Could you check a few things on this model? Use its own coordinates, in mm. A direction names the side the tool comes from. Coordinates: 2 decimals unless noted, no trailing zeros. Order: outer loops, then holes, each group sorted by start corner. A loop starts at its lowest first (then second) coordinate and runs counter-clockwise, first axis right, second up. Notation, with made-up numbers: (22.25, 33) -> (46.25, 33) arc R25 ccw to (46.25, 45) -> close; hole circle Ø11 at (-12.75, 86). An arc over 180 degrees is marked (long way). Use a Markdown table: item, result. Add a question column.
1) Will this pin go through, and if not, where does the flat tip stop? pin 1 Ø3 at (x, z) = (-2, -4.5) entering from -Y.
2) If we section it at C-C (z = 3.75): Write out the boundary of the cut face in (x, y), plus the area to 3 significant figures.
3) If I drill on L1, parallel to Y at x = 0.15, z = 0.5; L2, parallel to X at y = -0.1, z = 7; L3, parallel to Y at x = -1.7, z = 5.75, over which ranges is the centre line in solid material (lowest first)? Write a range as [from, to].
4) Which directions (+Z, -Z, +X, -X, +Y, -Y) give clear straight access to the entire face, cutting with the end or side of a thin tool? Please do faces 1 (the cylindrical face through (0, 2, 0)), 2 (the flat face through (1, -2, -10)), 3 (the flat face through (-1, 2, 10)).
5) Thinking about a two-plate mould opening in Z: for faces 4 (the conical face through (0.719, 0.938, 12.479)), 5 (the cylindrical face through (-3, 0, 0)), 6 (the conical face through (0.822, -0.428, 12.146)), which applies, +Z half, -Z half, draft (parallel to the pull), parting line (faces both ways), or undercut?
6) If we section it at A-A (x = 0): Write out the boundary of the cut face in (y, z).
Autodesk Inventor part; units mm, degrees
ref_plane "YZ Plane" through (0, 0, 0) normal (1, 0, 0) x (0, 1, 0)
ref_plane "XZ Plane" through (0, 0, 0) normal (0, 1, 0) x (-1, 0, 0)
ref_plane "XY Plane" through (0, 0, 0) normal (0, 0, 1) x (1, 0, 0)
sketch "Sketch1" plane through (0, 0, 0) normal (0, 0, 1) x (1, 0, 0)
  circle A0 centre (0, 0) radius 3
  circle A1 centre (0, 0) radius 2
  dimension "d0" = 6
  dimension "d1" = 4
extrude "Extrusion1" add sketch "Sketch1" along normal mid plane 20
sketch "Sketch2" plane through (0, 0, 0) normal (1, 0, 0) x (0, 1, 0)
  line L0 (3, 10) -> (-3, 10) construction
  line L1 (0, 10) -> (0, 13) construction
  line L2 (-3, -10) -> (-3, 10) construction
  line L3 (-3, 10) -> (-0.8, 13)
  line L4 (-0.8, 13) -> (-0.3, 13)
  line L5 (-0.3, 13) -> (-2.5, 10)
  line L6 (-3, 10) -> (-2.5, 10)
  point P0 (0, 0)
  point P1 (-0.55, 13)
  dimension "d4" = 3
  dimension "d6" = 0.3
  dimension "d7" = 0.5
revolve "Revolution1" add sketch "Sketch2" angle 360 about axis through (0, 0, 10) along (0, 0, 1)
properties part number "Nozzle"
Answer sheet:
| question | item | result |
|---|---|---|
| 1 | pin 1 | y = -2.96 |
| 2 | outline | circle Ø6 at (0, 0); hole circle Ø4 at (0, 0) |
| 2 | area | 15.7 mm2 |
| 3 | L1 | [-3, -1.99], [1.99, 3] |
| 3 | L2 | [-3, -2], [2, 3] |
| 3 | L3 | [-2.47, -1.05], [1.05, 2.47] |
| 4 | face 1 | -Z |
| 4 | face 2 | -Z, +X, -X, +Y, -Y |
| 4 | face 3 | none |
| 5 | face 4 | +Z half |
| 5 | face 5 | draft |
| 5 | face 6 | undercut |
| 6 | outline | (-3, -10) -> (-2, -10) -> (-2, 10) -> (-2.5, 10) -> (-0.3, 13) -> (-0.8, 13) -> (-3, 10) -> close; (0.3, 13) -> (2.5, 10) -> (2, 10) -> (2, -10) -> (3, -10) -> (3, 10) -> (0.8, 13) -> close |
